```python
from build123d import *

# Parameters (mm, degrees)
F0_R      = 1.15
F1_DEPTH  = 2
F2_DEPTH  = 105
F4_R      = 2.75
F4_R_2    = 1.75
F5_DEPTH  = 2
F6_DEPTH  = 2
F7_DEPTH  = 16
F9_R      = 1.15
F10_DEPTH = 18
F12_DEPTH = 2


with BuildPart() as f1:
    # F0 (on Top) → F1 (new body)
    with BuildSketch(Plane.XY):
        with BuildLine():
            ThreePointArc((0, 2.8), (0.8201010127, 0.8201010127), (2.8, 0))
            Line((2.8, 0), (84.2, 0))
            ThreePointArc((84.2, 0), (86.1798989873, 0.8201010127), (87, 2.8))
            Line((87, 2.8), (87, 53.2))
            ThreePointArc((87, 53.2), (86.1798989873, 55.1798989873), (84.2, 56))
            Line((84.2, 56), (2.8, 56))
            ThreePointArc((2.8, 56), (0.8201010127, 55.1798989873), (0, 53.2))
            Line((0, 53.2), (0, 2.8))
        make_face()
        with Locations((3.5, 3.5)):
            Circle(F0_R, mode=Mode.SUBTRACT)
        with Locations((61.5, 3.5)):
            Circle(F0_R, mode=Mode.SUBTRACT)
        with Locations((3.5, 52.5)):
            Circle(F0_R, mode=Mode.SUBTRACT)
        with Locations((61.5, 52.5)):
            Circle(F0_R, mode=Mode.SUBTRACT)
        with Locations((3.5, 3.5)):
            Circle(F0_R)
        with Locations((61.5, 52.5)):
            Circle(F0_R)
        with Locations((61.5, 3.5)):
            Circle(F0_R)
        with Locations((3.5, 52.5)):
            Circle(F0_R)
    extrude(amount=F1_DEPTH)

    # F0 (on Top) → F2 (join)
    with BuildSketch(Plane.XY):
        with Locations((61.5, 3.5)):
            Circle(F0_R)
        with Locations((61.5, 52.5)):
            Circle(F0_R)
        with Locations((3.5, 52.5)):
            Circle(F0_R)
        with Locations((3.5, 3.5)):
            Circle(F0_R)
    extrude(amount=F2_DEPTH)


with BuildPart() as f5:
    # F4 (on offset) → F5 (new body)
    with BuildSketch(Plane.XY.offset(25)):
        with BuildLine():
            Line((84.2, 56), (2.8, 56))
            ThreePointArc((2.8, 56), (0.8201010127, 55.1798989873), (0, 53.2))
            Line((0, 53.2), (0, 2.8))
            ThreePointArc((0, 2.8), (0.8201010127, 0.8201010127), (2.8, 0))
            Line((2.8, 0), (84.2, 0))
            ThreePointArc((84.2, 0), (86.1798989873, 0.8201010127), (87, 2.8))
            Line((87, 2.8), (87, 53.2))
            ThreePointArc((87, 53.2), (86.1798989873, 55.1798989873), (84.2, 56))
        make_face()
        with Locations((3.5, 3.5)):
            Circle(F4_R, mode=Mode.SUBTRACT)
        with Locations((61.5, 3.5)):
            Circle(F4_R, mode=Mode.SUBTRACT)
        with Locations((3.5, 52.5)):
            Circle(F4_R, mode=Mode.SUBTRACT)
        with Locations((61.5, 52.5)):
            Circle(F4_R, mode=Mode.SUBTRACT)
        with Locations((3.5, 3.5)):
            Circle(F4_R)
        with Locations((3.5, 3.5)):
            Circle(F4_R_2, mode=Mode.SUBTRACT)
        with Locations((61.5, 3.5)):
            Circle(F4_R)
        with Locations((61.5, 3.5)):
            Circle(F4_R_2, mode=Mode.SUBTRACT)
        with Locations((61.5, 52.5)):
            Circle(F4_R)
        with Locations((61.5, 52.5)):
            Circle(F4_R_2, mode=Mode.SUBTRACT)
        with Locations((3.5, 52.5)):
            Circle(F4_R)
        with Locations((3.5, 52.5)):
            Circle(F4_R_2, mode=Mode.SUBTRACT)
        with Locations((3.5, 3.5)):
            Circle(F4_R_2)
        with Locations((61.5, 3.5)):
            Circle(F4_R_2)
        with Locations((61.5, 52.5)):
            Circle(F4_R_2)
        with Locations((3.5, 52.5)):
            Circle(F4_R_2)
    extrude(amount=F5_DEPTH)

    # F4 (on offset) → F6 (join, through all)
    with BuildSketch(Plane.XY.offset(25)):
        with Locations((3.5, 3.5)):
            Circle(F4_R)
        with Locations((3.5, 3.5)):
            Circle(F4_R_2, mode=Mode.SUBTRACT)
        with Locations((3.5, 52.5)):
            Circle(F4_R)
        with Locations((3.5, 52.5)):
            Circle(F4_R_2, mode=Mode.SUBTRACT)
        with Locations((61.5, 52.5)):
            Circle(F4_R)
        with Locations((61.5, 52.5)):
            Circle(F4_R_2, mode=Mode.SUBTRACT)
        with Locations((61.5, 3.5)):
            Circle(F4_R)
        with Locations((61.5, 3.5)):
            Circle(F4_R_2, mode=Mode.SUBTRACT)
    extrude(amount=F6_DEPTH)

    # F4 (on offset) → F7 (join)
    with BuildSketch(Plane.XY.offset(25)):
        with Locations((3.5, 3.5)):
            Circle(F4_R)
        with Locations((3.5, 3.5)):
            Circle(F4_R_2, mode=Mode.SUBTRACT)
        with Locations((3.5, 52.5)):
            Circle(F4_R)
        with Locations((3.5, 52.5)):
            Circle(F4_R_2, mode=Mode.SUBTRACT)
        with Locations((61.5, 3.5)):
            Circle(F4_R)
        with Locations((61.5, 3.5)):
            Circle(F4_R_2, mode=Mode.SUBTRACT)
        with Locations((61.5, 52.5)):
            Circle(F4_R)
        with Locations((61.5, 52.5)):
            Circle(F4_R_2, mode=Mode.SUBTRACT)
    extrude(amount=-F7_DEPTH)

    # F9 (on face) → F10 (join)
    with BuildSketch(Plane.XY.offset(27)):
        with Locations((3.5, 52.5)):
            Circle(F9_R)
        with Locations((61.5, 52.5)):
            Circle(F9_R)
        with Locations((61.5, 3.5)):
            Circle(F9_R)
        with Locations((3.5, 3.5)):
            Circle(F9_R)
    extrude(amount=F10_DEPTH)

    # F11 (on face) → F12 (cut)
    with BuildSketch(Plane.XY.offset(27)):
        with BuildLine():
            Line((6.3, 46.8), (6.3, 9.2))
            ThreePointArc((6.3, 9.2), (7.1493903346, 7.1493903346), (9.2, 6.3))
            Line((9.2, 6.3), (77.8, 6.3))
            ThreePointArc((77.8, 6.3), (79.8506096654, 7.1493903346), (80.7, 9.2))
            Line((80.7, 9.2), (80.7, 46.8))
            ThreePointArc((80.7, 46.8), (79.8506096654, 48.8506096654), (77.8, 49.7))
            Line((77.8, 49.7), (9.2, 49.7))
            ThreePointArc((9.2, 49.7), (7.1493903346, 48.8506096654), (6.3, 46.8))
        make_face()
    extrude(amount=-F12_DEPTH, mode=Mode.SUBTRACT)


solid = f5.part
```
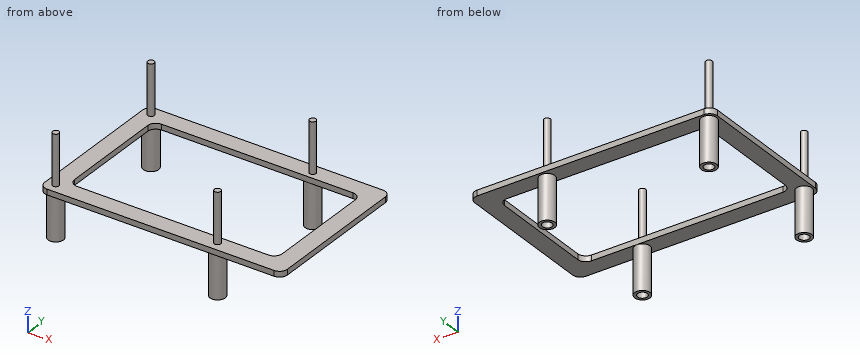
Can you work these out from the model? Positions are in its coordinate system, mm. Give positions to 0.01 mm unless a question says otherwise; leave off trailing zeros. Write each loop counter-clockwise with the first axis right and the second up, starting at its lowest first coordinate (ties: lowest second). Pieces come first, ordered by that corner, then holes. Notation, with made-up numbers: (-36, -38) -> (-11, -38) arc R7 cw to (-11, -26) -> close; hole circle Ø10 at (7, 61.25). An arc over 180 degrees is marked (long way). Write item = value, one per line.
(1) Suppose I cut it at C-C on y = 30. Write out the boundary of the cut face in (x, z), then the cut area to 3 significant figures.
Worked out:
outline = (0, 25) -> (6.3, 25) -> (6.3, 27) -> (0, 27) -> close; (80.7, 25) -> (87, 25) -> (87, 27) -> (80.7, 27) -> close
area = 25.2 mm^2
(2) Suppose I cut it at B-B on x = 35.5. Write out the boundary of the cut face in (y, z).
Worked out:
outline = (0, 25) -> (6.3, 25) -> (6.3, 27) -> (0, 27) -> close; (49.7, 25) -> (56, 25) -> (56, 27) -> (49.7, 27) -> close
(3) I'm going to push flat-ended pins straight in: P1, Ø3, axis at x = 3.5, y = 52.5, coming from the -Z side; P2, Ø12, axis at y = 33, z = 23, coming from the +X side; P3, Ø1.5, axis at x = 60, z = 21.5, coming from the -Y side. Where does each tip first touch, or does it pass through?
Worked out:
P1 = 25
P2 = 87
P3 = 0.85
(4) Suppose I cut it at A-A on z = 12. Write out the boundary of the cut face in (x, y).
Worked out:
outline = circle Ø5.5 at (3.5, 3.5); circle Ø5.5 at (3.5, 52.5); circle Ø5.5 at (61.5, 3.5); circle Ø5.5 at (61.5, 52.5); hole circle Ø3.5 at (3.5, 3.5); hole circle Ø3.5 at (3.5, 52.5); hole circle Ø3.5 at (61.5, 3.5); hole circle Ø3.5 at (61.5, 52.5)
(5) I need wall thicknesses on probe 1 along Y at (x, z) = (61.5, 19.5); probe 2 along Y at (x, z) = (59, 23); probe 3 along Z at (x, y) = (56, 3.5). Which ranges of each line are inside material? Lowest first, please. Write a range as from..to.
Worked out:
probe_1 = 0.75..1.75, 5.25..6.25, 49.75..50.75, 54.25..55.25
probe_2 = 2.35..4.65, 51.35..53.65
probe_3 = 25..27
(6) Suppose I cut it at D-D on z = 33. Write out the boundary of the cut face in (x, y).
Worked out:
outline = circle Ø2.3 at (3.5, 3.5); circle Ø2.3 at (3.5, 52.5); circle Ø2.3 at (61.5, 3.5); circle Ø2.3 at (61.5, 52.5)
